from build123d import *

# Parameters (mm, degrees)
SKETCH3_W          = 0.7874
SKETCH3_H          = 5.4356
CUT_EXTRUDE1_DEPTH = 1.1938


with BuildPart() as part:
    # Sketch2 → Revolve1 (revolve)
    with BuildSketch(Plane(origin=(0, 0, 0), x_dir=(1, 0, 0), z_dir=(0, 1, 0))):
        Polygon((0, 0), (15.875, 0), (17.653, -1.778), (-9.525, -1.778), (-9.525, 0.9398), (0, 0.9398), align=None)
    revolve(axis=Axis((-9.525, 0, 1.778), (1, 0, 0)))

    # Sketch3 → Cut-Extrude1 (cut)
    with BuildSketch(Plane.ZY.offset(9.525)):
        with Locations((1.778, 0)):
            Rectangle(SKETCH3_W, SKETCH3_H)
    extrude(amount=-CUT_EXTRUDE1_DEPTH, mode=Mode.SUBTRACT)


solid = part.part
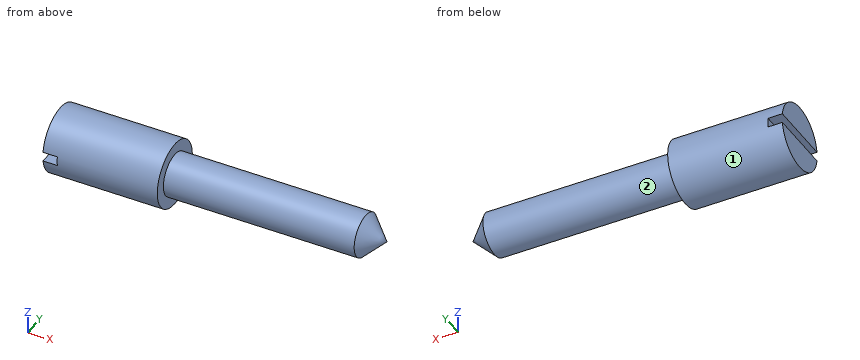
The model under review builds one solid part; all positions refer to its coordinate system, in mm. Face numbers are marked on the shaded views. A direction names the side the tool comes from. Round coordinates to 2 decimals unless told otherwise and drop trailing zeros. Order: outer loops, then holes, each group sorted by start corner. A loop starts at its lowest first (then second) coordinate and runs counter-clockwise, first axis right, second up. Notation, with made-up numbers: (-1.75, 20) -> (50.25, 20) arc R37 ccw to (50.25, 58) -> close; hole circle Ø6 at (69.5, -31). An arc over 180 degrees is marked (long way). Use CSV: the item, a comma, the result in double quotes. Start each with the question number.
(1) Consider section A-A on x = -3.5. Write out the cut boundary in (y, z).
(2) Insertion check: pin 1 (1.3 mm diameter, centred on x = -9, y = -1, fed in from +Z); pin 2 (1.5 mm diameter, centred on x = 3.5, z = 3.5, fed in from -Y); pin 3 (1.5 mm diameter, centred on y = -1, z = 4, fed in from +X). Each pin has a flat end and moves straight along its axis. Give the tip position at first contact, or say it passes through.
(3) Wall thickness on probe 1 along X at (y, z) = (-1.7, 0.45) (3 decimals); probe 2 along Y at (x, z) = (8, 1.75); probe 3 along Y at (x, z) = (4.75, 2.25): over which ranges is each line inside the solid? List them lowest first. Write a range as from..to.
(4) Consider section B-B on x = 10.75. Write out the cut boundary in (y, z).
(5) Tool access review of the marked faces 1 and 2: name each direction out of +Z, -Z, +X, -X, +Y, -Y from which nothing blocks a thin tool from reaching the whole face with its end or side.
Responses:
1,outline,"circle Ø5.44 at (0, 1.78)"
2,pin 1,"z = 4.47"
2,pin 2,"y = -1.49"
2,pin 3,"x = 15.97"
3,probe 1,"-9.525..0"
3,probe 2,"-1.78..1.78"
3,probe 3,"-1.71..1.71"
4,outline,"circle Ø3.56 at (0, 1.78)"
5,face 1,"+X, -X"
5,face 2,"+X"
